Autodesk Inventor part; units mm, degrees
ref_plane "YZ Plane" through (0, 0, 0) normal (1, 0, 0) x (0, 1, 0)
ref_plane "XZ Plane" through (0, 0, 0) normal (0, 1, 0) x (-1, 0, 0)
ref_plane "XY Plane" through (0, 0, 0) normal (0, 0, 1) x (1, 0, 0)
sketch "Sketch1" plane through (0, 0, 0) normal (0, 0, 1) x (1, 0, 0)
  line L0 (-225, -129) -> (225, -129)
  line L1 (225, -129) -> (225, 129)
  line L2 (225, 129) -> (-225, 129)
  line L3 (-225, 129) -> (-225, -129)
  line L4 (-225, -129) -> (225, 129) construction
  line L5 (225, -129) -> (-225, 129) construction
  point P0 (0, 0)
  dimension "d0" = 450
  dimension "d1" = 258
extrude "Extrusion1" add sketch "Sketch1" along normal mid plane 5
sketch "Sketch2" plane through (0, 0, 2.5) normal (0, 0, 1) x (1, 0, 0)
  circle A0 centre (-105.5, -99.5) radius 19.5 construction
  line L0 (-225, -129) -> (225, -129) construction
  line L1 (-225, 129) -> (-225, -129) construction
  circle A1 centre (-23.5, -99.5) radius 19.5 construction
  circle A2 centre (76.5, -99.5) radius 12.5 construction
  circle A3 centre (151.5, -99.5) radius 12.5 construction
  circle A4 centre (-191, 15) radius 24 construction
  circle A5 centre (-129, 15) radius 18 construction
  circle A6 centre (-78.5, 15) radius 12.5 construction
  circle A7 centre (-33.5, 15) radius 12.5 construction
  circle A8 centre (-191, 15) radius 16
  circle A9 centre (-129, 15) radius 12.5
  circle A10 centre (-78.5, 15) radius 8
  circle A11 centre (-33.5, 15) radius 8
  circle A12 centre (-105.5, -99.5) radius 14
  circle A13 centre (-23.5, -99.5) radius 14
  circle A14 centre (76.5, -99.5) radius 8
  circle A15 centre (151.5, -99.5) radius 8
  point P0 (0, 0)
  dimension "d4" = 39
  dimension "d5" = 29.5
  dimension "d6" = 119.5
  dimension "d7" = 39
  dimension "d8" = 25
  dimension "d9" = 25
  dimension "d10" = 48
  dimension "d11" = 36
  dimension "d12" = 25
  dimension "d13" = 25
  dimension "d14" = 29.5
  dimension "d15" = 29.5
  dimension "d16" = 29.5
  dimension "d17" = 144
  dimension "d18" = 144
  dimension "d19" = 144
  dimension "d20" = 144
  dimension "d21" = 82
  dimension "d22" = 100
  dimension "d23" = 75
  dimension "d24" = 34
  dimension "d25" = 62
  dimension "d26" = 50.5
  dimension "d27" = 45
  dimension "d28" = 32
  dimension "d29" = 25
  dimension "d30" = 16
  dimension "d31" = 16
  dimension "d32" = 28
  dimension "d33" = 28
  dimension "d34" = 16
  dimension "d35" = 16
extrude "Extrusion2" cut sketch "Sketch2" against normal blind 5
equation "\"d0\" = boxw"
equation "\"d1\" = boxh"
equation "\"d2\" = pvct"
equation "\"d4\" = waterouter"
equation "\"d6\" = 0.5 * waterouter + distsidewater"
equation "\"d7\" = airoutouter"
equation "\"d8\" = pumpouter"
equation "\"d9\" = pumpouter"
equation "\"d10\" = diaphouter"
equation "\"d11\" = diaetapeouter"
equation "\"d12\" = dialoadouter"
equation "\"d13\" = dialoadouter"
equation "\"d21\" = distbubblewater"
equation "\"d22\" = distpumpbubble"
equation "\"d23\" = distpumps"
equation "\"d28\" = diaph"
equation "\"d29\" = diaetape"
equation "\"d30\" = pumpinner"
equation "\"d31\" = pumpinner"
equation "\"d32\" = waterinner"
equation "\"d33\" = airoutinner"
equation "\"d34\" = pumpinner"
equation "\"d35\" = pumpinner"
equation "\"d36\" = pvct"
equation "\"solhole\" = 3"
equation "\"solholespacing\" = 16"
equation "\"ssolw\" = 63"
equation "\"bsoll\" = 126"
equation "\"bsolw\" = 91"
equation "\"bsolh\" = 126"
equation "\"tapl\" = 31"
equation "\"tl\" = 32"
equation "\"eloboww\" = 25"
equation "\"pvct\" = 5"
equation "\"boxw\" = 450"
equation "\"boxh\" = 258"
equation "\"supporth\" = 15"
equation "\"play\" = 0.5"
equation "\"pcbw\" = 76"
equation "\"arw\" = 54"
equation "\"pcbl\" = 86"
equation "\"arl\" = 102"
equation "\"psuh\" = 85"
equation "\"pcbh\" = 46"
equation "\"screenl\" = 115"
equation "\"screenw\" = 197"
equation "\"seph\" = 105"
equation "\"diapowerouter\" = 25"
equation "\"dialoadouter\" = 25"
equation "\"diaetapeouter\" = 36"
equation "\"diaphouter\" = 48"
equation "\"diaload\" = 16"
equation "\"diaetape\" = 25"
equation "\"diaph\" = 32"
equation "\"distbubblewater\" = 82"
equation "\"diapower\" = 16"
equation "\"distpumpbubble\" = 100"
equation "\"waterinner\" = 28"
equation "\"distpumps\" = 75"
equation "\"airoutouter\" = 39"
equation "\"airoutinner\" = 28"
equation "\"pumpouter\" = 25"
equation "\"waterouter\" = 39"
equation "\"pumpinner\" = 16"
equation "\"airinouter\" = 39"
equation "\"airininner\" = 28"
properties part number "sb_front_back" material "PVC-Piping"
Input: part model. Units: mm. Frame: model coordinates. Give positions to 0.01 mm unless a question says otherwise; leave off trailing zeros. Order: outer loops, then holes, each group sorted by start corner. A loop starts at its lowest first (then second) coordinate and runs counter-clockwise, first axis right, second up.
1. Cut plane C-C (z = 0.65). State how many separate pieces and enclosed holes the cut face has, and give its area (3 significant figures).
Computed:
separate pieces: 1
enclosed holes: 8
area: 113,000 mm2
2. Cut plane D-D (y = 15). Return loops of the section in (x, z).
Computed:
outline: (-225, -2.5) - (-207, -2.5) - (-207, 2.5) - (-225, 2.5) - close; (-175, -2.5) - (-141.5, -2.5) - (-141.5, 2.5) - (-175, 2.5) - close; (-116.5, -2.5) - (-86.5, -2.5) - (-86.5, 2.5) - (-116.5, 2.5) - close; (-70.5, -2.5) - (-41.5, -2.5) - (-41.5, 2.5) - (-70.5, 2.5) - close; (-25.5, -2.5) - (225, -2.5) - (225, 2.5) - (-25.5, 2.5) - close
3. Cut plane A-A (x = -191). Return loops of the section in (y, z).
Computed:
outline: (-129, -2.5) - (-1, -2.5) - (-1, 2.5) - (-129, 2.5) - close; (31, -2.5) - (129, -2.5) - (129, 2.5) - (31, 2.5) - close
4. Line query: probe 1 along Y at (x, z) = (-78.5, 0.15); probe 2 along Y at (x, z) = (-106, -0.55); probe 3 along X at (y, z) = (28, -0.2). Output: solid intervals per line, ascending.
Computed:
probe 1: y = -129 to 7, 23 to 129
probe 2: y = -129 to -113.49, -85.51 to 129
probe 3: x = -225 to -200.33, -181.67 to 225
5. Draft query along Y for faces 1 (the face through (70.151, -104.368, 0.035)), 2 (the face through (-3, 2, 2.5)). Return one class per face: released by +Y, released by -Y, zero draft, split by the parting line, or undercut.
Computed:
face 1: undercut
face 2: zero draft
6. Cut plane B-B (y = -99.5). Return loops of the section in (x, z), and give its area (3 significant figures).
Computed:
outline: (-225, -2.5) - (-119.5, -2.5) - (-119.5, 2.5) - (-225, 2.5) - close; (-91.5, -2.5) - (-37.5, -2.5) - (-37.5, 2.5) - (-91.5, 2.5) - close; (-9.5, -2.5) - (68.5, -2.5) - (68.5, 2.5) - (-9.5, 2.5) - close; (84.5, -2.5) - (143.5, -2.5) - (143.5, 2.5) - (84.5, 2.5) - close; (159.5, -2.5) - (225, -2.5) - (225, 2.5) - (159.5, 2.5) - close
area: 1,810 mm2
